Input: dimensioned drawing with shaded views. Units: mm. Origin: part minimum x, y, z. A direction names the side the tool comes from. Round coordinates to 2 decimals unless told otherwise and drop trailing zeros. Order: outer loops, then holes, each group sorted by start corner. A loop starts at its lowest first (then second) coordinate and runs counter-clockwise, first axis right, second up. Notation, with made-up numbers: (-7, -22.75) - (-3, -22.75) arc R7 ccw to (-3, -14.75) - close; hole circle Ø7 at (77.25, 3). An arc over 180 degrees is marked (long way). Return JSON: item names as keys, results as strings. Group by question number.
1) Mould query, pull axis Z, two halves, no side actions, for the marked faces 1, 2 and 3. Classes: pulls with the +Z half, pulls with the -Z half, needs draft (parallel to the pull), parting line crosses it, or undercut.
2) Ray query, line 1 (Z direction, x = 7, y = 44); line 2 (X direction, y = 10, z = 64.5); line 3 (X direction, y = 14, z = 32). Return the intervals inside material, ascending. Write a range as from..to.
3) Section B-B, the plane y = 35. Return loops of the section in (x, z).
4) Access query for the marked faces 4 and 5. Directions: +Z, -Z, +X, -X, +Y, -Y. A direction counts if a zero-diameter tool reaches every point of the face in a straight line with its end or side. Return the directions, or none.
5) Section A-A, the plane x = 9. Return loops of the section in (y, z), plus the area to 3 significant figures.
6) Section C-C, the plane z = 69.5. Return loops of the section in (x, y), plus the area to 3 significant figures.
7) Contact query for flat-ended pins moving along their axis: P1, Ø6, axis at y = 19.5, z = 25.5, coming from the -X side; P2, Ø7.5, axis at y = 53.5, z = 68, coming from the -X side; P3, Ø5, axis at y = 64, z = 18.5, coming from the -X side. Output: stop coordinate, or through.
8) Section D-D, the plane z = 41. Return loops of the section in (x, y).
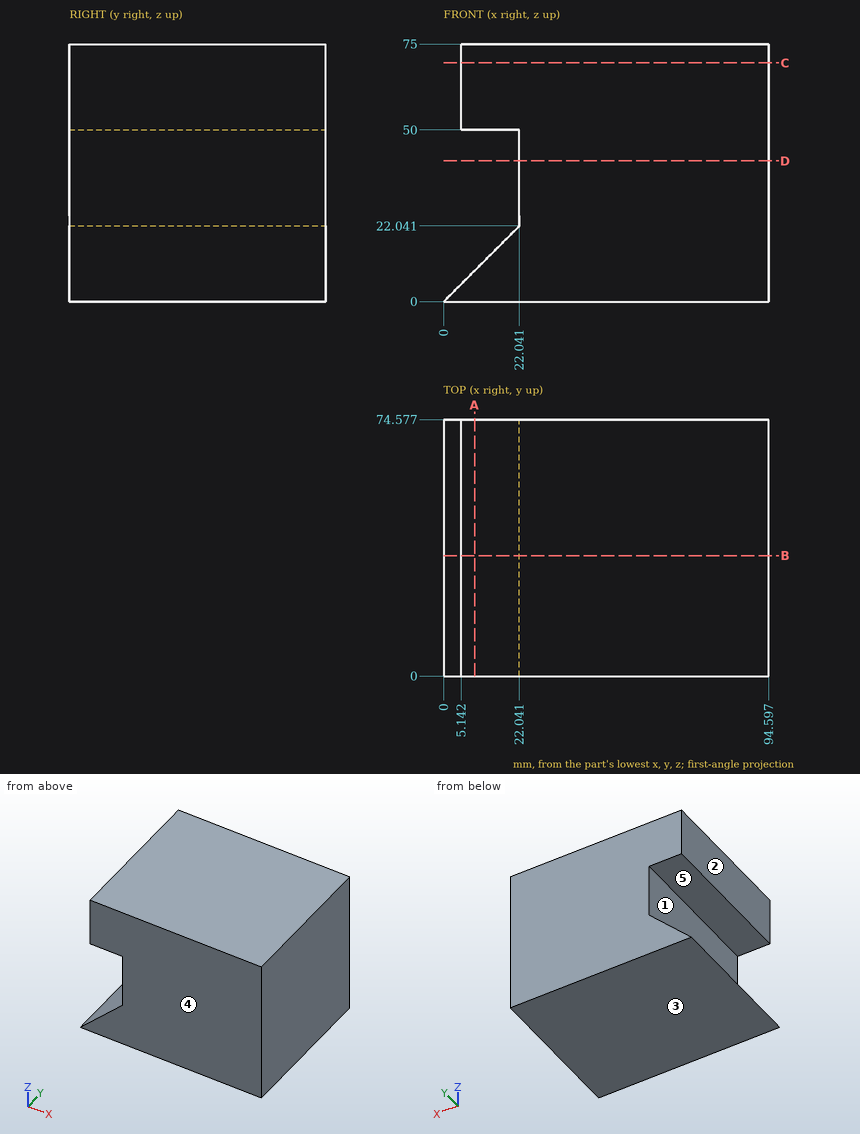
Geometry check:
{
 "1": {"face 1": "undercut", "face 2": "needs draft", "face 3": "pulls with the -Z half"},
 "2": {"line 1": "0..7, 50..75", "line 2": "5.14..94.6", "line 3": "22.04..94.6"},
 "3": {"outline": "(0, 0) - (94.6, 0) - (94.6, 75) - (5.14, 75) - (5.14, 50) - (22.04, 50) - (22.04, 22.04) - close"},
 "4": {"face 4": "+Z, -Z, +X, -X, -Y", "face 5": "-X, +Y, -Y"},
 "5": {"outline": "(0, 0) - (74.58, 0) - (74.58, 9) - (0, 9) - close; (0, 50) - (74.58, 50) - (74.58, 75) - (0, 75) - close", "area": "2,540 mm2"},
 "6": {"outline": "(5.14, 0) - (94.6, 0) - (94.6, 74.58) - (5.14, 74.58) - close", "area": "6,670 mm2"},
 "7": {"P1": "x = 22.04", "P2": "x = 5.14", "P3": "x = 16"},
 "8": {"outline": "(22.04, 0) - (94.6, 0) - (94.6, 74.58) - (22.04, 74.58) - close"}
}
